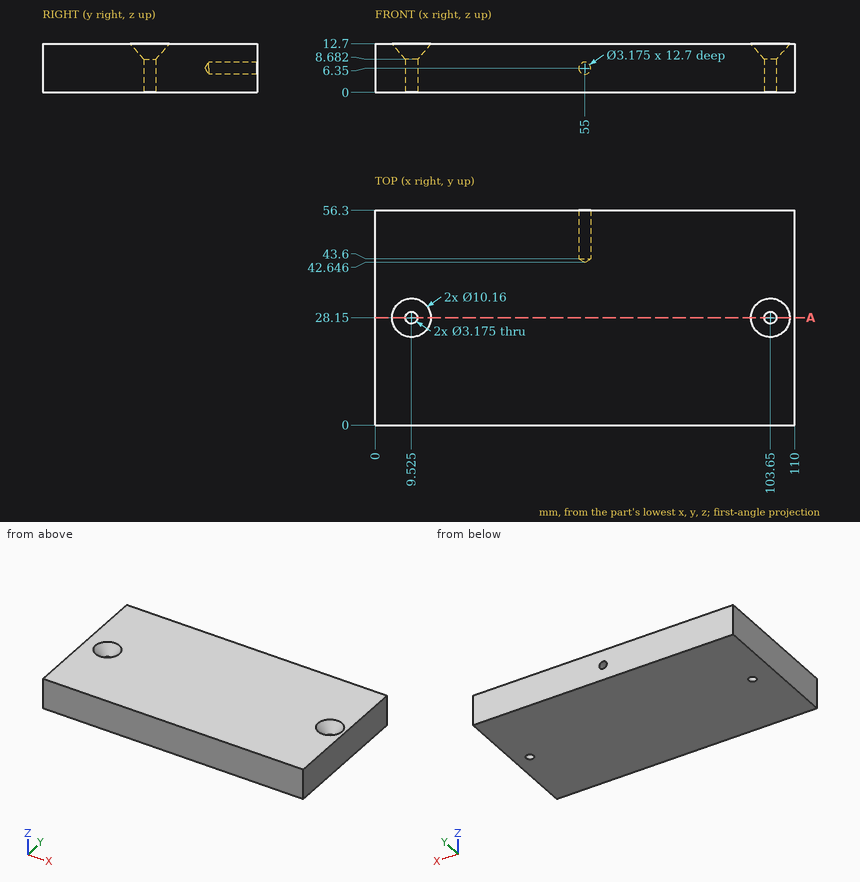
Geometry check sheet. Reference: drawing and pictorial views, mm from the part's lowest x, y, z. Coordinates: 2 decimals unless noted, no trailing zeros. Order: outer loops, then holes, each group sorted by start corner. A loop starts at its lowest first (then second) coordinate and runs counter-clockwise, first axis right, second up.
Item 1: Scan lines: line 1 along X through (y, z) = (28.15, 6); line 2 along Z through (x, y) = (55, 46); line 3 along Y through (x, z) = (103.65, 4.75). Record each from-to range of solid material in increasing order.
Item 2: Section check A-A (y = 28.15). Enter the section's corners in (x, z) (1 decimal), plus the area to 3 significant figures.
Item 3: Depth check by flat-ended pin: pin 1 (4 mm diameter, centred on x = 9.525, y = 28.15, fed in from -Z); pin 2 (3.5 mm diameter, centred on x = 103.65, y = 28.15, fed in from +Z). Enter the tip coordinate at first touch or a pass-through.
Check sheet entries:
1. line 1: x = 0 to 7.94, 11.11 to 102.06, 105.24 to 110
1. line 2: z = 0 to 4.76, 7.94 to 12.7
1. line 3: y = 0 to 26.56, 29.74 to 56.3
2. outline: (0, 0) - (7.9, 0) - (7.9, 8.7) - (4.4, 12.7) - (0, 12.7) - close; (11.1, 0) - (102.1, 0) - (102.1, 8.7) - (98.6, 12.7) - (14.6, 12.7) - (11.1, 8.7) - close; (105.2, 0) - (110, 0) - (110, 12.7) - (108.7, 12.7) - (105.2, 8.7) - close
2. area: 1,290 mm2
3. pin 1: stops at z = 0
3. pin 2: stops at z = 8.87
